Could you check a few things on this drawing? It's one solid part, dimensions in mm from its lowest x, y, z. A direction names the side the tool comes from. Round coordinates to 2 decimals unless told otherwise and drop trailing zeros. Write each loop counter-clockwise with the first axis right and the second up, starting at its lowest first coordinate (ties: lowest second). Pieces come first, ordered by that corner, then holes. Notation, with made-up numbers: (76, -33) - (94, -33) arc R22 ccw to (94, 1) - close; hole circle Ø3 at (26.5, 78). An arc over 180 degrees is marked (long way). Use one line per item in the form item = value. Start each with the question number.
1. We'd pull the mould along Y, two halves only. Please class the marked faces 4, 5 and 6: +Y half, -Y half, draft (parallel to the pull), parting line (faces both ways), or undercut.
2. I want a section at D-D, the plane z = 8.75. List the corners of the cut face in (x, y) for me, plus the area to 3 significant figures.
3. I want a section at C-C, the plane y = 58.5. List the corners of the cut face in (x, z) for me, plus the area to 3 significant figures.
4. Which directions (+Z, -Z, +X, -X, +Y, -Y) give clear straight access to the entire face, cutting with the end or side of a thin tool? Please do the marked faces 1, 2 and 3.
5. If I drill on line 1 along Y through (x, z) = (59.9, 5); line 2 along X through (y, z) = (52.5, 5.5); line 3 along X through (y, z) = (77, 6), over which ranges is the centre line in solid material (lowest first)?
6. I want a section at B-B, the plane x = 59.9. List the corners of the cut face in (y, z) for me, plus the area to 3 significant figures.
7. I want a section at A-A, the plane y = 5. List the corners of the cut face in (x, z) for me, plus the area to 3 significant figures.
8. Will these pins go through, and if not, where does the flat tip stop? pin 1 (4 mm diameter, centred on x = 23, z = 10.5, fed in from -Y); pin 2 (4 mm diameter, centred on x = 23, y = 63.5, fed in from +Z); pin 3 (3 mm diameter, centred on x = 33.5, z = 6, fed in from +Y); pin 4 (5 mm diameter, centred on x = 31.5, y = 78.5, fed in from +Z).
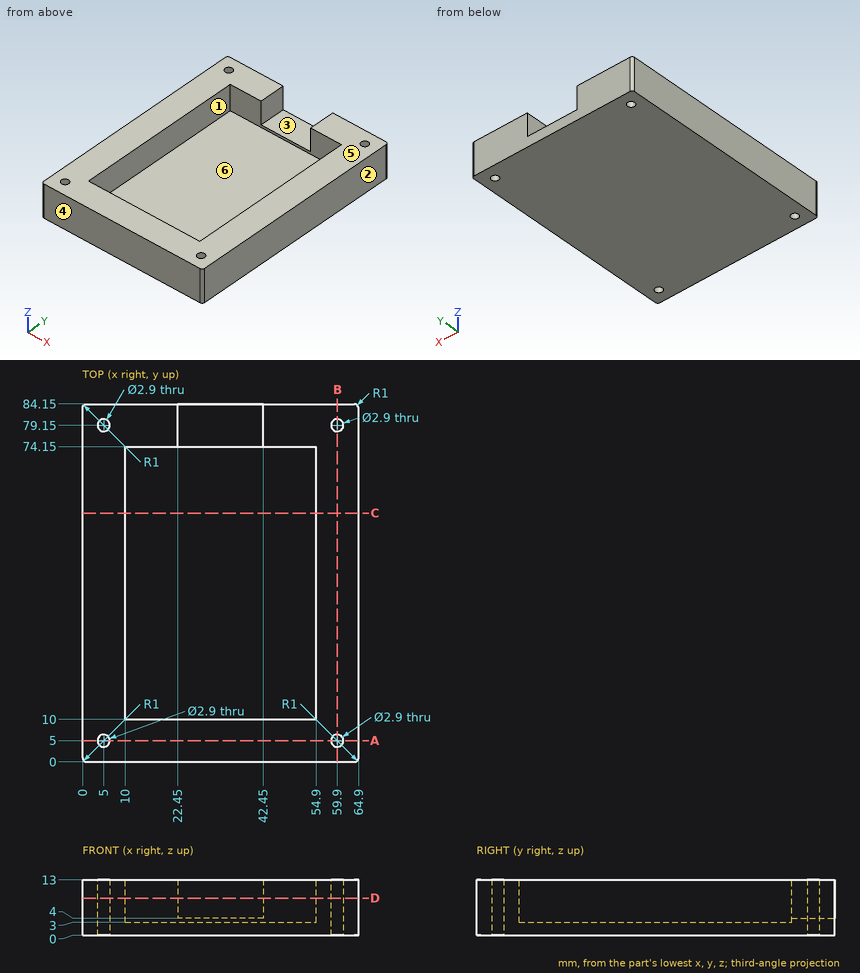
Model answer:
q1.face_4 = -Y half
q1.face_5 = draft
q1.face_6 = undercut
q2.outline = (0, 1) arc R1 ccw to (1, 0) - (63.9, 0) arc R1 ccw to (64.9, 1) - (64.9, 83.15) arc R1 ccw to (63.9, 84.15) - (42.45, 84.15) - (42.45, 74.15) - (54.9, 74.15) - (54.9, 10) - (10, 10) - (10, 74.15) - (22.45, 74.15) - (22.45, 84.15) - (1, 84.15) arc R1 ccw to (0, 83.15) - close; hole circle Ø2.9 at (5, 5); hole circle Ø2.9 at (5, 79.15); hole circle Ø2.9 at (59.9, 5); hole circle Ø2.9 at (59.9, 79.15)
q2.area = 2,350 mm2
q3.outline = (0, 0) - (64.9, 0) - (64.9, 13) - (54.9, 13) - (54.9, 3) - (10, 3) - (10, 13) - (0, 13) - close
q3.area = 395 mm2
q4.face_1 = +Z
q4.face_2 = +Z, -Z, +X, +Y, -Y
q4.face_3 = +Z, +Y
q5.line_1 = 0 to 3.55, 6.45 to 77.7, 80.6 to 84.15
q5.line_2 = 0 to 10, 54.9 to 64.9
q5.line_3 = 0 to 22.45, 42.45 to 64.9
q6.outline = (0, 0) - (3.55, 0) - (3.55, 13) - (0, 13) - close; (6.45, 0) - (77.7, 0) - (77.7, 13) - (6.45, 13) - close; (80.6, 0) - (84.15, 0) - (84.15, 13) - (80.6, 13) - close
q6.area = 1,020 mm2
q7.outline = (0, 0) - (3.55, 0) - (3.55, 13) - (0, 13) - close; (6.45, 0) - (58.45, 0) - (58.45, 13) - (6.45, 13) - close; (61.35, 0) - (64.9, 0) - (64.9, 13) - (61.35, 13) - close
q7.area = 768 mm2
q8.pin_1 = 0
q8.pin_2 = 3
q8.pin_3 = 10
q8.pin_4 = 4
